Could you check a few things on this model? Use its own coordinates, in mm. A direction names the side the tool comes from. Give positions to 0.01 mm unless a question says otherwise; leave off trailing zeros. Order: outer loops, then holes, each group sorted by start corner. A loop starts at its lowest first (then second) coordinate and runs counter-clockwise, first axis right, second up. Notation, with made-up numbers: (83, 3) -> (119, 3) arc R24 cw to (119, 38) -> close; hole circle Ø7 at (-1, -36). An arc over 180 degrees is marked (long way). Answer as CSV lines item,"result". Start each with the question number.
(1) I need wall thicknesses on L1, parallel to Y at x = -31.5, z = -70; L2, parallel to Z at x = 5.5, y = -24.5; L3, parallel to Y at x = -20.5, z = -63. Which ranges of each line are inside material? Lowest first, please.
(2) On a 3-axis mill with a long thin cutter (end or side, diameter ignored), from which of +Z, -Z, +X, -X, +Y, -Y can I reach the whole of each face in a straight line? I mean faces 1 (the face through (-1, 0, -69)), 2 (the face through (39.291, 0, -50)), 3 (the face through (-1, 7.5, -50)), 4 (the face through (-1, -23, -25)). Say none if no direction works.
(3) Will these pins go through, and if not, where does the flat tip stop? pin 1 Ø8 at (y, z) = (-12, -46) entering from +X; pin 2 Ø7.5 at (y, z) = (-1, -42) entering from -X; pin 3 Ø3 at (x, z) = (19, -71) entering from -Y; pin 4 Ø1.8 at (x, y) = (-4, 0) entering from -Z.
(4) We'd pull the mould along X, two halves only. Please class faces 5 (the face through (26.603, 0.105, -35.784)), 6 (the face through (-1, 3, -72)), 7 (the face through (-39.291, 0, -50)): released by +X, released by -X, zero draft, split by the parting line, or undercut.
(5) I want a section at D-D (z = -52). Please give me the cut outline in (x, y), plus the area to 3 significant figures.
(6) I want a section at B-B (y = 0). Please give me the cut outline in (x, z), plus the area to 3 significant figures.
(7) I want a section at C-C (x = 0). Please give me the cut outline in (y, z), plus the area to 3 significant figures.
(8) I want a section at A-A (z = -40). Please give me the cut outline in (x, y), plus the area to 3 significant figures.
```python
from build123d import *

# Parameters (mm, degrees)
F0_R        = 40
F1_DEPTH    = 25
F2_W        = 78.5811682275
F2_H        = 15
F3_DEPTH    = 50
F4_W        = 6
F4_H        = 12
F5_DEPTH    = 79.2915841138
F6_R        = 5
F7_DEPTH    = 25
F8_T4_DEPTH = 78.5811682275
F8_S5_R     = 40
F8_T6_DEPTH = 41


# Not quite as in the source:
# - a fillet or chamfer that OpenCascade refuses, or shapes differently, is made with other operations: its cross-section is extruded or revolved along the edge and cut away or added


with BuildPart() as f1:
    # F0 (on Top) → F1 (new body)
    with BuildSketch(Plane.XY):
        Circle(F0_R)
    extrude(amount=-F1_DEPTH)

    # F2 (on face) → F3 (join)
    with BuildSketch(Plane(origin=(0, 0, -25), x_dir=(1, 0, 0), z_dir=(0, 0, -1))):
        Rectangle(F2_W, F2_H)
    extrude(amount=F3_DEPTH)

    # F4 (on face) → F5 (cut, through all)
    with BuildSketch(Plane(origin=(-39.2905841138, 0, 0), x_dir=(0, -1, 0), z_dir=(-1, 0, 0))):
        with Locations((0, -75)):
            Rectangle(F4_W, F4_H)
    extrude(amount=-F5_DEPTH, mode=Mode.SUBTRACT)

    # F6 (on face) → F7 (cut)
    with BuildSketch(Plane(origin=(0, 7.5, 0), x_dir=(-1, 0, 0), z_dir=(0, 1, 0))):
        with Locations((-29.2905841138, -40)):
            Circle(F6_R)
        with Locations((29.2905841138, -40)):
            Circle(F6_R)
    extrude(amount=-F7_DEPTH, mode=Mode.SUBTRACT)

    # F8: fillet of radius 5 on 2 edges, made by hand


with BuildPart() as f8_tool2:
    # F8_s3 → F8_t4 (new body)
    with BuildSketch(Plane.YZ.offset(39.2905841138)):
        with BuildLine():
            ThreePointArc((-12.5, -25), (-8.9644660941, -26.4644660941), (-7.5, -30))
            Line((-7.5, -30), (-7.5, -25))
            Line((-7.5, -25), (-12.5, -25))
        make_face()
    extrude(amount=-F8_T4_DEPTH)

    # F8_s5 → F8_t6 (intersect, symmetric)
    with BuildSketch(Plane.XY.offset(-27.5)):
        Circle(F8_S5_R)
    extrude(amount=F8_T6_DEPTH, both=True, mode=Mode.INTERSECT)


with BuildPart() as f1_1:
    add(f1.part)

    # F8_t1: union F8_tool2
    add(f8_tool2.part)

    # F8_s7 → F8_t8 (revolve, cut)
    with BuildSketch(Plane.XZ):
        with BuildLine():
            ThreePointArc((40, -5), (38.5355339059, -1.4644660941), (35, 0))
            Line((35, 0), (40, 0))
            Line((40, 0), (40, -5))
        make_face()
    revolve(axis=Axis((0, 0, 0), (0, 0, 1)), mode=Mode.SUBTRACT)


solid = f1_1.part
```
Final values:
1,L1,"-7.5 to -3, 3 to 7.5"
1,L2,"-25 to 0"
1,L3,"-7.5 to 7.5"
2,face 1,"-Z, +X, -X"
2,face 2,"-Z, +X, +Y, -Y"
2,face 3,"-Z, +X, -X, +Y"
2,face 4,"-Z, +X, -X, -Y"
3,pin 1,"through"
3,pin 2,"x = -39.29"
3,pin 3,"y = -7.5"
3,pin 4,"z = -69"
4,face 5,"undercut"
4,face 6,"zero draft"
4,face 7,"released by -X"
5,outline,"(-39.29, -7.5) -> (39.29, -7.5) -> (39.29, 7.5) -> (-39.29, 7.5) -> close"
5,area,"1,180 mm²"
6,outline,"(-40, -25) -> (-39.29, -25) -> (-39.29, -69) -> (39.29, -69) -> (39.29, -25) -> (40, -25) -> (40, -5) arc R5 ccw to (35, 0) -> (-35, 0) arc R5 ccw to (-40, -5) -> close; hole circle Ø10 at (-29.29, -40); hole circle Ø10 at (29.29, -40)"
6,area,"5,290 mm²"
7,outline,"(-40, -25) -> (-12.5, -25) arc R5 cw to (-7.5, -30) -> (-7.5, -75) -> (-3, -75) -> (-3, -69) -> (3, -69) -> (3, -75) -> (7.5, -75) -> (7.5, -25) -> (40, -25) -> (40, -5) arc R5 ccw to (35, 0) -> (-35, 0) arc R5 ccw to (-40, -5) -> close"
7,area,"2,710 mm²"
8,outline,"(-39.29, -7.5) -> (-34.29, -7.5) -> (-34.29, 7.5) -> (-39.29, 7.5) -> close; (-24.29, -7.5) -> (24.29, -7.5) -> (24.29, 7.5) -> (-24.29, 7.5) -> close; (34.29, -7.5) -> (39.29, -7.5) -> (39.29, 7.5) -> (34.29, 7.5) -> close"
8,area,"879 mm²"
